from build123d import *

# Parameters (mm, degrees)
F0_W     = 38.8
F0_H     = 38.8
F0_R     = 18
F1_DEPTH = 38.5
F2_DEPTH = 16
F3_R     = 1.164619
F3_R_2   = 1.25
F4_DEPTH = 3


with BuildPart() as f1:
    # F0 (on Front) → F1 (new body)
    with BuildSketch(Plane.XZ):
        Rectangle(F0_W, F0_H)
        Circle(F0_R, mode=Mode.SUBTRACT)
        Circle(F0_R)
    extrude(amount=-F1_DEPTH)

    # F0 (on Front) → F2 (join)
    with BuildSketch(Plane.XZ):
        Circle(F0_R)
    extrude(amount=F2_DEPTH)

    # F3 (on face) → F4 (cut)
    with BuildSketch(Plane.XY.offset(19.4)):
        with Locations((12.5, 2.5)):
            Circle(F3_R)
        with Locations((-12.5, 2.5)):
            Circle(F3_R_2)
    extrude(amount=-F4_DEPTH, mode=Mode.SUBTRACT)


solid = f1.part
Geometry: final body of the model. Coordinates: model frame, mm. A direction names the side the tool comes from. Give positions to 0.01 mm unless a question says otherwise; leave off trailing zeros. Order: outer loops, then holes, each group sorted by start corner. A loop starts at its lowest first (then second) coordinate and runs counter-clockwise, first axis right, second up. Notation, with made-up numbers: (64, 58) -> (116, 58) arc R6 cw to (116, 64) -> close; hole circle Ø7 at (88.5, -16.75). An arc over 180 degrees is marked (long way). Put each result on its own line as item: value.
Q1. Pin query (flat end, axial travel): pin 1 (1.2 mm diameter, centred on x = -12.5, y = 2.5, fed in from +Z); pin 2 (2 mm diameter, centred on x = -11, y = -2.5, fed in from -Z). Return the tip coordinate at first contact, or that it passes through.
Here are the results:
pin 1: stops at z = 16.4
pin 2: stops at z = -14.97
Q2. Draft query along X for faces 1 (the face through (-19.4, 19, 0)), 2 (the face through (19.4, 19, 0)), 3 (the face through (-13, 3, 16.4)), 4 (the face through (0, 38.5, 0)). Return one class per face: released by +X, released by -X, zero draft, split by the parting line, or undercut.
Here are the results:
face 1: released by -X
face 2: released by +X
face 3: undercut
face 4: zero draft
Q3. Section B-B, the plane z = 0. Return loops of the section in (x, y), then the cut area to 3 significant figures.
Here are the results:
outline: (-19.4, 0) -> (-18, 0) -> (-18, -16) -> (18, -16) -> (18, 0) -> (19.4, 0) -> (19.4, 38.5) -> (-19.4, 38.5) -> close
area: 2,070 mm^2
Q4. Material intervals for L1, parallel to Y at x = -12.5, z = 18.15; L2, parallel to Y at x = -12, z = 18; L3, parallel to Y at x = 12, z = -14.5, sorted ascending.
Here are the results:
L1: y = 0 to 1.25, 3.75 to 38.5
L2: y = 0 to 1.35, 3.65 to 38.5
L3: y = 0 to 38.5
Q5. Section C-C, the plane y = -9.5. Return loops of the section in (x, z).
Here are the results:
outline: circle Ø36 at (0, 0)
Q6. Reachability of faces 5 (the face through (-2.343, -7.888, 17.847)), 6 (the face through (-13.421, 3.345, 17.921)), 7 (the face through (0, 19, -19.4)) from +Z, -Z, +X, -X, +Y, -Y: full face, straight path, thin tool, end or side. Return the list, or none.
Here are the results:
face 5: -Y
face 6: +Z
face 7: -Z, +X, -X, +Y, -Y
Q7. Section A-A, the plane x = 0. Return loops of the section in (y, z), then the cut area to 3 significant figures.
Here are the results:
outline: (-16, -18) -> (0, -18) -> (0, -19.4) -> (38.5, -19.4) -> (38.5, 19.4) -> (0, 19.4) -> (0, 18) -> (-16, 18) -> close
area: 2,070 mm^2
Q8. Section D-D, the plane x = -12.5. Return loops of the section in (y, z).
Here are the results:
outline: (-16, -12.95) -> (0, -12.95) -> (0, -19.4) -> (38.5, -19.4) -> (38.5, 19.4) -> (3.75, 19.4) -> (3.75, 16.4) -> (1.25, 16.4) -> (1.25, 19.4) -> (0, 19.4) -> (0, 12.95) -> (-16, 12.95) -> close
